Here's how the part is built. I have some questions about the finished solid (model axes, mm). Face numbers are marked on the shaded views. A direction names the side the tool comes from. Give positions to 0.01 mm unless a question says otherwise; leave off trailing zeros. Write each loop counter-clockwise with the first axis right and the second up, starting at its lowest first coordinate (ties: lowest second). Pieces come first, ordered by that corner, then holes. Notation, with made-up numbers: (66, 40) - (114, 40) arc R22 ccw to (114, 58) - close; hole circle Ø3 at (78.25, 89). An arc over 180 degrees is marked (long way). One line per item, written item: value. Start each with the question number.
1) Imagine slicing it at A-A on z = 29.75. Write out the boundary of the cut face in (x, y) (3 decimals).
2) Imagine slicing it at D-D on x = 5. Write out the boundary of the cut face in (y, z) (3 decimals).
3) Please list where these lines run through material, in increasing order: L1, parallel to X at y = -0.9, z = 8.75 (3 decimals); L2, parallel to Z at x = 1.85, y = -34.25; L3, parallel to Y at x = 1.2, z = 10. Write a range as [from, to].
4) Imagine slicing it at C-C on z = 21. Write out the boundary of the cut face in (x, y), plus the area to 3 significant figures.
5) I'm going to push flat-ended pins straight in: P1, Ø5, axis at x = 0.5, y = -18.5, coming from the +Z side; P2, Ø8, axis at y = -17.5, z = 31, coming from the -X side; P3, Ø3, axis at x = -5.5, z = 10, coming from the +Y side; P4, Ø1, axis at y = -35, z = 18.5, coming from the -X side. Where does each tip first touch, or does it pass through?
6) On a 3-axis mill with a long thin cutter (end or side, diameter ignored), from which of +Z, -Z, +X, -X, +Y, -Y can I reach the whole of each face in a straight line? I mean the marked faces 4, 5, 6, 7 and 8. Say none if no direction works.
7) Imagine slicing it at B-B on x = -10. Write out the boundary of the cut face in (y, z), plus the area to 3 significant figures.
8) We'd pull the mould along X, two halves only. Please class the marked faces 1, 2 and 3: +X half, -X half, draft (parallel to the pull), parting line (faces both ways), or undercut.
from build123d import *

# Parameters (mm, degrees)
EXTRUDE_1_DEPTH         = 35.5
SKETCH_2_W              = 29.5
SKETCH_2_H              = 39
CUT_EXTRUDE_2_DEPTH     = 15
SKETCH_3_W              = 3
SKETCH_3_H              = 30.64
CUT_EXTRUDE_3_DEPTH     = 3
SKETCH_4_R              = 0.8
CUT_EXTRUDE_4_DEPTH     = 3
SKETCH_5_R              = 1.075
SKETCH_5_R_2            = 4
CUT_EXTRUDE_6_DEPTH     = 4
SKETCH2_W               = 29.5
SKETCH2_H               = 42
BOSS_EXTRUDE1_DEPTH     = 22
CUT_EXTRUDE1_DEPTH      = 58.482606065
SKETCH4_W               = 17
SKETCH4_H               = 42
CUT_EXTRUDE2_DEPTH      = 22
SKETCH5_R               = 0.8
CUT_EXTRUDE3_DEPTH      = 6
CUT_EXTRUDE4_DEPTH      = 58.482606065
CUT_EXTRUDE4_DEPTH_BACK = 58.482606065
CUT_EXTRUDE5_DEPTH      = 57.282415378
CUT_EXTRUDE5_DEPTH_BACK = 57.282415378
CUT_EXTRUDE6_DEPTH      = 57.282415378
CUT_EXTRUDE6_DEPTH_BACK = 57.282415378
CUT_EXTRUDE7_DEPTH      = 57.073612332
CUT_EXTRUDE7_DEPTH_BACK = 57.073612332
SKETCH9_W               = 7.089051245
SKETCH9_H               = 1.624595939
CUT_EXTRUDE8_DEPTH      = 53.697841512
CUT_EXTRUDE8_DEPTH_BACK = 53.697841512
SKETCH11_W              = 2.8
SKETCH11_H              = 2.8
CUT_EXTRUDE9_DEPTH      = 58.864064842
CUT_EXTRUDE10_DEPTH     = 57.073612332
SKETCH13_W              = 6.25
SKETCH13_H              = 1.804834364
CUT_EXTRUDE11_DEPTH     = 1.647183607
FILLET1_R               = 10
FILLET2_R               = 9


with BuildPart() as part:
    # 草图1 → 凸台-拉伸1 (new body)
    with BuildSketch(Plane.XY):
        Polygon((0, 0), (18, 0), (18, -3), (3, -11.36), (3, -42), (0, -42), align=None)
    extrude(amount=EXTRUDE_1_DEPTH)

    # 草图2 → 切除-拉伸2 (cut)
    with BuildSketch(Plane(origin=(18, 0, 0), x_dir=(0, 0, -1), z_dir=(1, 0, 0))):
        with Locations((-17.75, -22.5)):
            Rectangle(SKETCH_2_W, SKETCH_2_H)
    extrude(amount=-CUT_EXTRUDE_2_DEPTH, mode=Mode.SUBTRACT)

    # 草图3 → 切除-拉伸3 (cut)
    with BuildSketch(Plane(origin=(0, 0, 0), x_dir=(0, 0, -1), z_dir=(1, 0, 0))):
        with Locations((-34, -26.68)):
            Rectangle(SKETCH_3_W, SKETCH_3_H)
        with Locations((-1.5, -26.68)):
            Rectangle(SKETCH_3_W, SKETCH_3_H)
    extrude(amount=CUT_EXTRUDE_3_DEPTH, mode=Mode.SUBTRACT)

    # 草图4 → 切除-拉伸4 (cut)
    with BuildSketch(Plane(origin=(0, 0, 0), x_dir=(0, 0, -1), z_dir=(1, 0, 0))):
        with Locations((-10, -17.25)):
            Circle(SKETCH_4_R)
        with Locations((-10, -34.25)):
            Circle(SKETCH_4_R)
        with Locations(Location((-25.5, -34.25, 0), (0, 0, 180))):
            Circle(SKETCH_4_R)
        with Locations(Location((-25.5, -17.25, 0), (0, 0, 180))):
            Circle(SKETCH_4_R)
    extrude(amount=CUT_EXTRUDE_4_DEPTH, mode=Mode.SUBTRACT)

    # 草图5 → 切除-拉伸6 (cut)
    with BuildSketch(Plane(origin=(0, 0, 0), x_dir=(1, 0, 0), z_dir=(0, 1, 0))):
        with Locations(Location((14, -17.75, 0), (0, 0, 270))):
            Circle(SKETCH_5_R)
        with Locations(Location((13.656854249, -23.406854249, 0), (0, 0, 270))):
            Circle(SKETCH_5_R)
        with Locations(Location((14, -29.75, 0), (0, 0, 270))):
            Circle(SKETCH_5_R)
        with Locations(Location((5, -26.75, 0), (0, 0, 270))):
            Circle(SKETCH_5_R)
        with Locations(Location((5, -8.75, 0), (0, 0, 270))):
            Circle(SKETCH_5_R)
        with Locations(Location((14, -5.75, 0), (0, 0, 270))):
            Circle(SKETCH_5_R)
        with Locations(Location((13.656854249, -12.093145751, 0), (0, 0, 270))):
            Circle(SKETCH_5_R)
        with Locations(Location((8, -17.75, 0), (0, 0, 270))):
            Circle(SKETCH_5_R_2)
        with Locations(Location((8, -23.75, 0), (0, 0, 270))):
            Circle(SKETCH_5_R)
        with Locations(Location((8, -11.75, 0), (0, 0, 270))):
            Circle(SKETCH_5_R)
        with Locations(Location((11, -26.75, 0), (0, 0, 270))):
            Circle(SKETCH_5_R)
        with Locations(Location((11, -8.75, 0), (0, 0, 270))):
            Circle(SKETCH_5_R)
        with Locations(Location((8, -29.75, 0), (0, 0, 270))):
            Circle(SKETCH_5_R)
        with Locations(Location((8, -5.75, 0), (0, 0, 270))):
            Circle(SKETCH_5_R)
    extrude(amount=-CUT_EXTRUDE_6_DEPTH, mode=Mode.SUBTRACT)

    # Sketch2 → Boss-Extrude1 (add)
    with BuildSketch(Plane.ZY):
        with Locations((17.75, -21)):
            Rectangle(SKETCH2_W, SKETCH2_H)
    extrude(amount=BOSS_EXTRUDE1_DEPTH)

    # Sketch3 → Cut-Extrude1 (cut, through all)
    with BuildSketch(Plane.XY.offset(32.5)):
        Polygon((0, -42), (-22, -11.36), (-22, -42), align=None)
    extrude(amount=-CUT_EXTRUDE1_DEPTH, mode=Mode.SUBTRACT)

    # Sketch4 → Cut-Extrude2 (cut)
    with BuildSketch(Plane.ZY.offset(22)):
        with Locations((17.75, -21)):
            Rectangle(SKETCH4_W, SKETCH4_H)
    extrude(amount=-CUT_EXTRUDE2_DEPTH, mode=Mode.SUBTRACT)

    # Sketch5 → Cut-Extrude3 (cut)
    with BuildSketch(Plane(origin=(-19.89820704, -14.287224376, 0), x_dir=(0, 0, 1), z_dir=(-0.8122979693681996, -0.5832426673009267, 0))):
        with Locations(Location((7.25, -7.719412775, 0), (0, 0, 270))):
            Circle(SKETCH5_R)
        with Locations(Location((7.25, -19.719412775, 0), (0, 0, 270))):
            Circle(SKETCH5_R)
        with Locations(Location((28.25, -7.719412775, 0), (0, 0, 270))):
            Circle(SKETCH5_R)
        with Locations(Location((28.25, -19.719412775, 0), (0, 0, 270))):
            Circle(SKETCH5_R)
    extrude(amount=-CUT_EXTRUDE3_DEPTH, mode=Mode.SUBTRACT)

    # Sketch6 → Cut-Extrude4 (cut, two sides: drawn at the far end of the back side and taken through both)
    with BuildSketch(Plane.XY.offset(32.5).offset(-CUT_EXTRUDE4_DEPTH_BACK)):
        Polygon((-18.640286498, -16.039164622), (0, -2.655146902), (0, 0), (-22, 0), (-22, -11.36), align=None)
    extrude(amount=CUT_EXTRUDE4_DEPTH + CUT_EXTRUDE4_DEPTH_BACK, mode=Mode.SUBTRACT)

    # Sketch7 → Cut-Extrude5 (cut, two sides: drawn at the far end of the back side and taken through both)
    with BuildSketch(Plane.XY.offset(32.5).offset(-CUT_EXTRUDE5_DEPTH_BACK)):
        Polygon((-5.922565911, -33.751480932), (0, -33.751480932), (0, -42), align=None)
    extrude(amount=CUT_EXTRUDE5_DEPTH + CUT_EXTRUDE5_DEPTH_BACK, mode=Mode.SUBTRACT)

    # Sketch8 → Cut-Extrude6 (cut, two sides: drawn at the far end of the back side and taken through both)
    with BuildSketch(Plane.XY.offset(32.5).offset(-CUT_EXTRUDE6_DEPTH_BACK)):
        Polygon((-16.735484956, -18.69203368), (-15.397481057, -17.731325919), (-17.302282599, -15.078456862), (-18.640286498, -16.039164622), align=None)
        Polygon((-13.97434516, -22.537548377), (-12.636341261, -21.576840617), (-8.798133161, -26.922417715), (-10.13613706, -27.883125476), align=None)
        Polygon((-7.089051245, -32.126884993), (-5.798120087, -31.199976198), (-3.966099716, -33.751480932), (-5.922565911, -33.751480932), align=None)
    extrude(amount=CUT_EXTRUDE6_DEPTH + CUT_EXTRUDE6_DEPTH_BACK, mode=Mode.SUBTRACT)

    # Sketch9 → Cut-Extrude7 (cut, two sides: drawn at the far end of the back side and taken through both)
    with BuildSketch(Plane.XY.offset(32.5).offset(-CUT_EXTRUDE7_DEPTH_BACK)):
        with Locations((-3.544525623, -32.939182962)):
            Rectangle(SKETCH9_W, SKETCH9_H)
    extrude(amount=CUT_EXTRUDE7_DEPTH + CUT_EXTRUDE7_DEPTH_BACK, mode=Mode.SUBTRACT)

    # Sketch10 → Cut-Extrude8 (cut, two sides: drawn at the far end of the back side and taken through both)
    with BuildSketch(Plane.XY.offset(9.25).offset(-CUT_EXTRUDE8_DEPTH_BACK)):
        Polygon((-10.059859583, -19.854018926), (0, -19.854018926), (0, -13.95755501), (0, -2.655146902), (-17.302282599, -15.078456862), (-15.397481057, -17.731325919), align=None)
    extrude(amount=CUT_EXTRUDE8_DEPTH + CUT_EXTRUDE8_DEPTH_BACK, mode=Mode.SUBTRACT)

    # Sketch11 → Cut-Extrude9 (cut, through all)
    with BuildSketch(Plane.ZY):
        with Locations((10, -17.25)):
            Rectangle(SKETCH11_W, SKETCH11_H)
        with Locations((25.5, -17.25)):
            Rectangle(SKETCH11_W, SKETCH11_H)
    extrude(amount=CUT_EXTRUDE9_DEPTH, mode=Mode.SUBTRACT)

    # Sketch12 → Cut-Extrude10 (cut, through all)
    with BuildSketch(Plane.XY.offset(32.5)):
        Polygon((-5.798120087, -31.199976198), (0, -31.199976198), (0, -32.126884993), (-9.163402462, -32.126884993), (-9.163402462, -31.199976198), align=None)
    extrude(amount=-CUT_EXTRUDE10_DEPTH, mode=Mode.SUBTRACT)

    # Sketch13 → Cut-Extrude11 (cut)
    with BuildSketch(Plane(origin=(-19.89820704, -14.287224376, 0), x_dir=(0, 0, 1), z_dir=(-0.8122979693681996, -0.5832426673009267, 0))):
        with Locations((6.125, -17.63999577)):
            Rectangle(SKETCH13_W, SKETCH13_H)
        with Locations((29.375, -17.63999577)):
            Rectangle(SKETCH13_W, SKETCH13_H)
    extrude(amount=-CUT_EXTRUDE11_DEPTH, mode=Mode.SUBTRACT)

    # Fillet1
    fillet1_edges = [part.edges().sort_by_distance(p)[0] for p in [
        (-10.059859583, -19.854018926, 6.125),
    ]]
    fillet(fillet1_edges, radius=FILLET1_R)

    # Fillet2
    fillet2_edges = [part.edges().sort_by_distance(p)[0] for p in [
        (-10.059859583, -19.854018926, 29.375),
    ]]
    fillet(fillet2_edges, radius=FILLET2_R)


solid = part.part
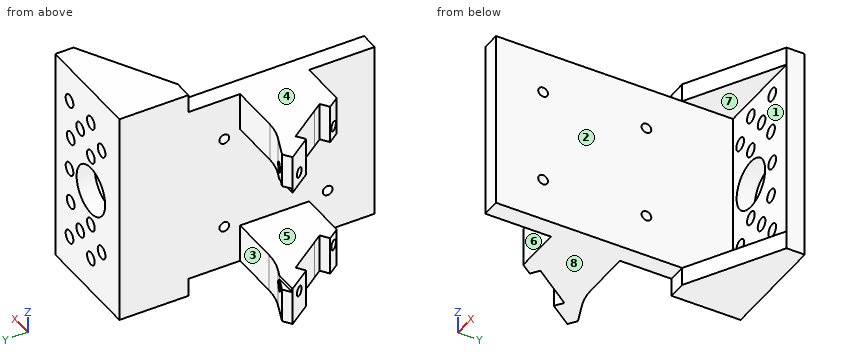
Numbers:
1. outline: (-16.735, -18.692) - (-13.974, -22.538) - (-12.636, -21.577) - (-7.745, -28.388) - (-9.083, -29.349) - (-7.755, -31.2) - (0, -31.2) - (0, -42) - (3, -42) - (3, -3) - (6.925, -3) - (6.925, 0) - (0, 0) - (0, -19.854) - (-8.336, -19.854) arc R9 cw to (-11.662, -19.217) - (-15.397, -17.731) - close; (9.075, -3) - (12.925, -3) - (12.925, 0) - (9.075, 0) - close; (15.075, -3) - (18, -3) - (18, 0) - (15.075, 0) - close
2. outline: (-10.245, 0) - (0, 0) - (0, 7.675) - (-3, 7.675) - (-3, 3) - (-10.245, 3) - close; (-10.245, 32.5) - (-3, 32.5) - (-3, 27.825) - (0, 27.825) - (0, 35.5) - (-10.245, 35.5) - close; (-3, 9.825) - (0, 9.825) - (0, 15.104) - (-3, 15.104) - close; (-3, 20.396) - (0, 20.396) - (0, 25.675) - (-3, 25.675) - close
3. L1: [0, 3.925], [6.075, 9.925], [12.075, 18]
3. L2: [3, 9.2], [10.8, 24.7], [26.3, 32.5]
3. L3: [-42, -35.05], [-33.45, -18.05], [-16.45, 0]
4. outline: (0, -42) - (3, -42) - (3, -3) - (5.67, -3) - (5.67, 0) - (0, 0) - close; (10.33, -3) - (18, -3) - (18, 0) - (10.33, 0) - close
4. area: 157 mm^2
5. P1: z = 32.5
5. P2: x = -16.74
5. P3: y = -19.85
5. P4: x = 0
6. face 4: +Z, +X, -X, -Y
6. face 5: -X, +Y, -Y
6. face 6: +Z, -Z, -X, -Y
6. face 7: +X, -Y
6. face 8: -Z, +X, -X, -Y
7. outline: (-25.25, 3) - (-19.68, 3) - (-19.68, 9.25) - (-25.25, 9.25) - close; (-25.25, 26.25) - (-19.7, 26.25) - (-19.7, 32.5) - (-25.25, 32.5) - close
7. area: 69.5 mm^2
8. face 1: draft
8. face 2: +X half
8. face 3: undercut
